Read the model definition and answer for the solid it produces. Units are mm, in the model's axes. A direction names the side the tool comes from. Coordinates: 2 decimals unless noted, no trailing zeros. Write each loop counter-clockwise with the first axis right and the second up, starting at its lowest first coordinate (ties: lowest second). Pieces come first, ordered by that corner, then holes. Notation, with made-up numbers: (67, 2) - (124, 2) arc R21 ccw to (124, 23) - close; hole circle Ø5 at (-3, 84). An arc over 180 degrees is marked (long way). Return JSON: item names as keys, results as strings.
```python
from build123d import *

# Parameters (mm, degrees)
SKETCH1_W               = 40
SKETCH1_H               = 50
BOSS_EXTRUDE1_DEPTH     = 2
SKETCH3_W               = 40
SKETCH3_H               = 6
CUT_EXTRUDE3_DEPTH      = 3
SKETCH8_W               = 40
SKETCH8_H               = 6
CUT_EXTRUDE4_DEPTH      = 10
BOSS_EXTRUDE2_DEPTH     = 10
CUT_EXTRUDE5_START      = 10
SKETCH9_R               = 6
CUT_EXTRUDE5_DEPTH      = 10
MIRROR4_START           = 10
MIRROR4_COPY_1_SKETCH_R = 6
MIRROR4_COPY_1_DEPTH    = 10
FILLET1_R               = 1.1


with BuildPart() as part:
    # Sketch1 → Boss-Extrude1 (new body)
    with BuildSketch(Plane.XY):
        with Locations((20, 25)):
            Rectangle(SKETCH1_W, SKETCH1_H)
    extrude(amount=BOSS_EXTRUDE1_DEPTH)

    # Sketch3 → Cut-Extrude3 (cut)
    with BuildSketch(Plane.XY.offset(2)):
        with Locations((20, 3)):
            Rectangle(SKETCH3_W, SKETCH3_H)
    extrude(amount=-CUT_EXTRUDE3_DEPTH, mode=Mode.SUBTRACT)

    # Sketch8 → Cut-Extrude4 (cut)
    with BuildSketch(Plane.XY.offset(2)):
        with Locations((20, 47)):
            Rectangle(SKETCH8_W, SKETCH8_H)
    extrude(amount=-CUT_EXTRUDE4_DEPTH, mode=Mode.SUBTRACT)

    # Sketch6 → Boss-Extrude2 (add, symmetric)
    with BuildSketch(Plane(origin=(20, 0, -40), x_dir=(0, 0, 1), z_dir=(-1, 0, 0))):
        with BuildLine():
            Line((43.77260129, 11.571238192), (44.515067527, 9.714158794))
            ThreePointArc((44.515067527, 9.714158794), (48.242796258, 9.312078644), (50, 6))
            ThreePointArc((50, 6), (46, 2), (42, 6))
            Line((42, 6), (40, 6))
            ThreePointArc((40, 6), (46, 0), (52, 6))
            ThreePointArc((52, 6), (49.364194387, 10.968117966), (43.77260129, 11.571238192))
        make_face()
    boss_extrude2 = extrude(amount=BOSS_EXTRUDE2_DEPTH, both=True)

    # Mirror2: Boss-Extrude2 across plane
    add(boss_extrude2.mirror(Plane(origin=(0, 25, 0), x_dir=(0, 0, 1), z_dir=(0, -1, 0))))

    # Sketch9 → Cut-Extrude5 (cut)
    with BuildSketch(Plane.ZY.offset(-10).offset(CUT_EXTRUDE5_START)):
        with Locations((6, 6)):
            Circle(SKETCH9_R)
    cut_extrude5 = extrude(amount=-CUT_EXTRUDE5_DEPTH, mode=Mode.SUBTRACT)

    # Mirror3: Cut-Extrude5 across plane
    add(cut_extrude5.mirror(Plane(origin=(20, 0, 0), x_dir=(0, 0, 1), z_dir=(1, 0, 0))), mode=Mode.SUBTRACT)

    # Mirror4: Cut-Extrude5 across plane
    add(cut_extrude5.mirror(Plane(origin=(0, 25, 0), x_dir=(0, 0, 1), z_dir=(0, -1, 0))), mode=Mode.SUBTRACT)

    # Mirror4 copy 1 sketch → Mirror4 copy 1 (cut)
    with BuildSketch(Plane(origin=(30, 50, 0), x_dir=(0, 0, 1), z_dir=(1, 0, 0)).offset(MIRROR4_START)):
        with Locations((6, 6)):
            Circle(MIRROR4_COPY_1_SKETCH_R)
    extrude(amount=-MIRROR4_COPY_1_DEPTH, mode=Mode.SUBTRACT)

    # Fillet1
    # the kernel refuses this fillet: 1.1 mm, written as the material it takes off along each edge
    with BuildSketch(Plane(origin=(70.828558189, 6, 0), x_dir=(0, 0.9192771195538384, 0.393610946830494), z_dir=(-1, 0, 0)), Plane(origin=(10, 6, 0), x_dir=(0, 0.9192771195538384, 0.3936109468304938), z_dir=(-1, 0, 0))) as fillet1_piece_1:
        with BuildLine():
            CenterArc((5.156303403, 1.011204832), FILLET1_R, 113.179370495, 133.641259009)
            Line((4.723331362, 2.022409663), (4.714671921, 2.04263376))
            Line((4.714671921, 2.04263376), (-0.008659441, 0.020224097))
            Line((-0.008659441, 0.020224097), (0.008659441, -0.020224097))
            ThreePointArc((0.008659441, -0.020224097), (2.361665681, 0.462337283), (4.714671921, -0.020224097))
            Line((4.714671921, -0.020224097), (4.723331362, 0))
        make_face()
    extrude(amount=40.828558189, mode=Mode.SUBTRACT)
    with BuildSketch(Plane(origin=(70.828558189, 6, 0), x_dir=(0, 0.9192771195538384, 0.393610946830494), z_dir=(-1, 0, 0))) as fillet1_piece_2_section:
        with BuildLine():
            CenterArc((5.156303403, 1.011204832), FILLET1_R, 113.179370495, 133.641259009)
            Line((4.723331362, 2.022409663), (4.714671921, 2.04263376))
            Line((4.714671921, 2.04263376), (-0.008659441, 0.020224097))
            Line((-0.008659441, 0.020224097), (0.008659441, -0.020224097))
            ThreePointArc((0.008659441, -0.020224097), (2.361665681, 0.462337283), (4.714671921, -0.020224097))
            Line((4.714671921, -0.020224097), (4.723331362, 0))
        make_face()
    fillet1_piece_2 = extrude(amount=71.657116378, mode=Mode.PRIVATE)
    fillet1_piece_2 = split(fillet1_piece_2, bisect_by=Plane(origin=(10, 9.140941458, 0.431936904), z_dir=(-1, 0, 0)), keep=Keep.TOP, mode=Mode.PRIVATE)
    add(fillet1_piece_2, mode=Mode.SUBTRACT)
    with BuildSketch(Plane(origin=(70.828558189, 44, 0), x_dir=(0, -0.9192771195538351, 0.39361094683050163), z_dir=(-1, 0, 0)), Plane(origin=(10, 44, 0), x_dir=(0, -0.9192771195538407, 0.39361094683048864), z_dir=(-1, 0, 0))) as fillet1_piece_3:
        with BuildLine():
            CenterArc((5.156303403, -1.011204832), FILLET1_R, 113.179370495, 133.641259009)
            Line((4.723331362, -2.022409663), (4.714671921, -2.04263376))
            Line((4.714671921, -2.04263376), (-0.008659441, -0.020224097))
            Line((-0.008659441, -0.020224097), (0.008659441, 0.020224097))
            ThreePointArc((0.008659441, 0.020224097), (2.361665681, -0.462337283), (4.714671921, 0.020224097))
            Line((4.714671921, 0.020224097), (4.723331362, 0))
        make_face()
    extrude(amount=40.828558189, mode=Mode.SUBTRACT)
    with BuildSketch(Plane(origin=(70.828558189, 44, 0), x_dir=(0, -0.9192771195538351, 0.39361094683050163), z_dir=(-1, 0, 0))) as fillet1_piece_4_section:
        with BuildLine():
            CenterArc((5.156303403, -1.011204832), FILLET1_R, 113.179370495, 133.641259009)
            Line((4.723331362, -2.022409663), (4.714671921, -2.04263376))
            Line((4.714671921, -2.04263376), (-0.008659441, -0.020224097))
            Line((-0.008659441, -0.020224097), (0.008659441, 0.020224097))
            ThreePointArc((0.008659441, 0.020224097), (2.361665681, -0.462337283), (4.714671921, 0.020224097))
            Line((4.714671921, 0.020224097), (4.723331362, 0))
        make_face()
    fillet1_piece_4 = extrude(amount=71.657116378, mode=Mode.PRIVATE)
    fillet1_piece_4 = split(fillet1_piece_4, bisect_by=Plane(origin=(10, 40.859058542, 0.431936904), z_dir=(-1, 0, 0)), keep=Keep.TOP, mode=Mode.PRIVATE)
    add(fillet1_piece_4, mode=Mode.SUBTRACT)
    with BuildSketch(Plane(origin=(40.828558189, 6, 0), x_dir=(0, 0.9192771195538384, 0.393610946830494), z_dir=(-1, 0, 0))) as fillet1_piece_5_section:
        with BuildLine():
            CenterArc((5.156303403, 1.011204832), FILLET1_R, 113.179370495, 133.641259009)
            Line((4.723331362, 2.022409663), (4.714671921, 2.04263376))
            Line((4.714671921, 2.04263376), (-0.008659441, 0.020224097))
            Line((-0.008659441, 0.020224097), (0.008659441, -0.020224097))
            ThreePointArc((0.008659441, -0.020224097), (2.361665681, 0.462337283), (4.714671921, -0.020224097))
            Line((4.714671921, -0.020224097), (4.723331362, 0))
        make_face()
    fillet1_piece_5 = extrude(amount=71.657116378, mode=Mode.PRIVATE)
    fillet1_piece_5 = split(fillet1_piece_5, bisect_by=Plane(origin=(30, 9.140941458, 0.431936904), z_dir=(1, 0, 0)), keep=Keep.TOP, mode=Mode.PRIVATE)
    add(fillet1_piece_5, mode=Mode.SUBTRACT)
    with BuildSketch(Plane(origin=(40.828558189, 44, 0), x_dir=(0, -0.9192771195538353, 0.3936109468305011), z_dir=(-1, 0, 0))) as fillet1_piece_6_section:
        with BuildLine():
            CenterArc((5.156303403, -1.011204832), FILLET1_R, 113.179370495, 133.641259009)
            Line((4.723331362, -2.022409663), (4.714671921, -2.04263376))
            Line((4.714671921, -2.04263376), (-0.008659441, -0.020224097))
            Line((-0.008659441, -0.020224097), (0.008659441, 0.020224097))
            ThreePointArc((0.008659441, 0.020224097), (2.361665681, -0.462337283), (4.714671921, 0.020224097))
            Line((4.714671921, 0.020224097), (4.723331362, 0))
        make_face()
    fillet1_piece_6 = extrude(amount=71.657116378, mode=Mode.PRIVATE)
    fillet1_piece_6 = split(fillet1_piece_6, bisect_by=Plane(origin=(30, 40.859058542, 0.431936904), z_dir=(1, 0, 0)), keep=Keep.TOP, mode=Mode.PRIVATE)
    add(fillet1_piece_6, mode=Mode.SUBTRACT)


solid = part.part
```
(1) Determine the mould class of faces 1 (the face through (20, 25, 2)), 2 (the face through (30, 47, 9)), 3 (the face through (5.07, 39.88, 0.68)) for opening direction Z: +Z half, -Z half, draft (parallel to the pull), parting line (faces both ways), or undercut.
Answer:
{"face 1": "undercut", "face 2": "draft", "face 3": "parting line"}
(2) Straight lines are drawn through the part: line 1 (Y direction, x = 22, z = 6); line 2 (Z direction, x = 21, y = 6); line 3 (Y direction, x = 11, z = 2.5). For each, find the intervals that lie inside material, in ascending order. Write a range as from..to.
Answer:
{"line 1": "0..2, 10..12, 38..40, 48..50", "line 2": "0..2, 10..12", "line 3": "1.13..4.06, 45.94..48.87"}
(3) A cutting plane is placed at A-A (z = 6). Determine the outline of the cut face in (x, y).
Answer:
{"outline": "(10, 0) - (30, 0) - (30, 2) - (10, 2) - close; (10, 10) - (30, 10) - (30, 12) - (10, 12) - close; (10, 38) - (30, 38) - (30, 40) - (10, 40) - close; (10, 48) - (30, 48) - (30, 50) - (10, 50) - close"}
(4) Which of the six approach directions +Z, -Z, +X, -X, +Y, -Y give full straight-line access (tool end or side, diameter ignored) to faces 4 (the face through (35.07, 39.88, 0.68)), 5 (the face through (5.07, 10.134, 0.651)), 6 (the face through (35.07, 10.134, 0.651)), 7 (the face through (20, 11, 4)), 8 (the face through (0, 25, 1))?
Answer:
{"face 4": "+X, +Y", "face 5": "-X, -Y", "face 6": "+X, -Y", "face 7": "+X, -X", "face 8": "+Z, -Z, -X, +Y, -Y"}
(5) Flat-ended cylindrical pins translate along their axes: P1, Ø5, axis at x = 29, z = 7, coming from the -Y side; P2, Ø6.5, axis at y = 6, z = 6, coming from the -X side; P3, Ø8, axis at x = 13.5, y = 12, coming from the +Z side; P4, Ø3.5, axis at y = 6.5, z = 8.5, coming from the -X side. Find the tip coordinate at first contact, or state that the pin passes through.
Answer:
{"P1": "y = 0", "P2": "through", "P3": "z = 11.66", "P4": "x = 10"}
(6) A cutting plane is placed at D-D (z = 8.5). Determine the outline of the cut face in (x, y).
Answer:
{"outline": "(10, 0.55) - (30, 0.55) - (30, 2.88) - (10, 2.88) - close; (10, 9.12) - (30, 9.12) - (30, 11.45) - (10, 11.45) - close; (10, 38.55) - (30, 38.55) - (30, 40.88) - (10, 40.88) - close; (10, 47.12) - (30, 47.12) - (30, 49.45) - (10, 49.45) - close"}
(7) A cutting plane is placed at C-C (x = 21). Determine the outline of the cut face in (y, z).
Answer:
{"outline": "(6, 0) - (44, 0) arc R6 ccw (long way) to (38.43, 3.77) - (40.29, 4.52) arc R4 cw (long way) to (44, 2) - (6, 2) arc R4 cw (long way) to (9.71, 4.52) - (11.57, 3.77) arc R6 ccw (long way) to start"}
(8) A cutting plane is placed at B-B (y = 5). Determine the outline of the cut face in (x, z).
Answer:
{"outline": "(10, 0.08) - (30, 0.08) - (30, 2.13) - (10, 2.13) - close; (10, 9.87) - (30, 9.87) - (30, 11.92) - (10, 11.92) - close"}
